```python
from build123d import *

# Parameters (mm, degrees)
FILLET1_R           = 1
CHAMFER1_SIZE       = 0.5
CHAMFER2_SIZE       = 0.5
SKETCH2_R           = 4.1
BOSS_EXTRUDE1_DEPTH = 15


# Read off the part's stored shape, not the designer's step: M8x1.0 Machine Threads Stud1
with BuildPart() as part:
    # Sketch1 → Revolve1 (revolve)
    with BuildSketch(Plane.XY, mode=Mode.PRIVATE) as revolve1_sk:
        Polygon((0, 0), (0, -7.5), (30, -7.5), (30, -9), (76, -9), (76, -5), (91, -5), (91, 0), align=None)
    revolve(revolve1_sk.sketch.rotate(Axis((0, 0, 0), (1, 0, 0)), 270), axis=Axis((0, 0, 0), (1, 0, 0)))

    # Fillet1
    fillet1_edges = [part.edges().sort_by_distance(p)[0] for p in [
        (76, 0, -5),
        (30, 0, -7.5),
    ]]
    fillet(fillet1_edges, radius=FILLET1_R)

    # Chamfer1
    chamfer1_edges = [part.edges().sort_by_distance(p)[0] for p in [
        (0, 0, -7.5),
    ]]
    chamfer(chamfer1_edges, length=CHAMFER1_SIZE)

    # Chamfer2
    chamfer2_edges = [part.edges().sort_by_distance(p)[0] for p in [
        (91, 0, -5),
        (76, 0, -9),
    ]]
    chamfer(chamfer2_edges, length=CHAMFER2_SIZE)

    # Sketch2 → Boss-Extrude1 (add)
    with BuildSketch(Plane(origin=(91, 0, 0), x_dir=(0, 0, -1), z_dir=(1, 0, 0))):
        Circle(SKETCH2_R)
    extrude(amount=BOSS_EXTRUDE1_DEPTH)

    # M8x1.0 Machine Threads Stud1 outline → M8x1.0 Machine Threads Stud1 (revolve, cut)
    with BuildSketch(Plane.YX):
        with BuildLine():
            ThreePointArc((3, 91.4), (3.117157288, 91.117157288), (3.4, 91))
            Line((3.4, 91), (4.1, 91))
            Line((4.1, 91), (4.1, 106))
            Line((4.1, 106), (3.4455, 106))
            Line((3.4455, 106), (4, 105.4455))
            Line((4, 105.4455), (4, 93.939230485))
            Line((4, 93.939230485), (3.053589838, 92.3))
            ThreePointArc((3.053589838, 92.3), (3.013629669, 92.203527618), (3, 92.1))
            Line((3, 92.1), (3, 91.4))
        make_face()
    revolve(axis=Axis((0, 0, 0), (1, 0, 0)), mode=Mode.SUBTRACT)


solid = part.part
```
The listing builds one solid part. Answer for the finished solid, in the listing's coordinates (mm). A direction names the side the tool comes from. Coordinates: 2 decimals unless noted, no trailing zeros. Write each loop counter-clockwise with the first axis right and the second up, starting at its lowest first coordinate (ties: lowest second). Pieces come first, ordered by that corner, then holes. Notation, with made-up numbers: (-40, 12.25) - (10, 12.25) arc R22 ccw to (10, 28.25) - close; hole circle Ø5 at (44, -25). An arc over 180 degrees is marked (long way). Return JSON: item names as keys, results as strings. Group by question number.
Q1. The part is cut by section A-A on x = 88. Write down the section's boundary in (y, z), and give its area (3 significant figures).
Q2. For a pull along X with two mould halves and no side action, classify faces 4 (the flat face through (76, 2, -6)), 5 (the cylindrical face through (91.7, -3, 0.1)), 6 (the flat face through (91, -3, -2)), 7 (the cylindrical face through (99.612, -0.867, -3.905)) as +X half, -X half, draft (parallel to the pull), parting line (faces both ways), or undercut.
Q3. Flat-ended cylindrical pins translate along their axes: pin 1 Ø6 at (x, y) = (20, 1) entering from -Z; pin 2 Ø3 at (x, y) = (90.5, 6) entering from -Z; pin 3 Ø10 at (x, z) = (75.5, -5.5) entering from -Y. Find the tip coordinate at first contact, or state that the pin passes through.
Q4. Find the intervals of material crossed by line 1 along X through (y, z) = (0.5, 6); line 2 along X through (y, z) = (1.25, -3); line 3 along X through (y, z) = (-0.5, 4.25), in increasing order. Write a range as [from, to].
Q5. The part is cut by section B-B on x = 11. Write down the section's boundary in (y, z), and give its area (3 significant figures).
Q6. Which of the six approach directions +Z, -Z, +X, -X, +Y, -Y give full straight-line access (tool end or side, diameter ignored) to faces 1 (the cylindrical face through (53.068, -2.703, 8.584)), 2 (the cylindrical face through (83.84, 4.88, -1.08)), 3 (the cylindrical face through (14.95, -0.33, -7.493))?
Evaluation:
{
 "1": {"outline": "circle Ø10 at (0, 0)", "area": "78.5 mm2"},
 "2": {"face 4": "+X half", "face 5": "undercut", "face 6": "undercut", "face 7": "draft"},
 "3": {"pin 1": "stops at z = -7.5", "pin 2": "stops at z = -2.18", "pin 3": "stops at y = -8.99"},
 "4": {"line 1": "x = [0, 76]", "line 2": "x = [0, 91.03], [92.64, 106]", "line 3": "x = [0, 91]"},
 "5": {"outline": "circle Ø15 at (0, 0)", "area": "177 mm2"},
 "6": {"face 1": "+X, -X", "face 2": "+X", "face 3": "-X"}
}
